from build123d import *

# Parameters (mm, degrees)
BOSS_EXTRUDE1_DEPTH     = 22.225
CUT_EXTRUDE3_DEPTH      = 155.828053821
CUT_EXTRUDE3_DEPTH_BACK = 155.828053821
BOSS_EXTRUDE3_DEPTH     = 12.7
SKETCH10_W              = 31.75
SKETCH10_H              = 3.175
CUT_EXTRUDE5_DEPTH      = 12.7
CUT_EXTRUDE4_REACH      = 158.104
SKETCH9_R               = 3.175
BOSS_EXTRUDE6_DEPTH     = 3.175
CUT_EXTRUDE8_REACH      = 139.445
BOSS_EXTRUDE7_DEPTH     = 12.7


with BuildPart() as part:
    # Sketch1 → Boss-Extrude1 (new body)
    with BuildSketch(Plane(origin=(0, 0, 0), x_dir=(1, 0, 0), z_dir=(0, 1, 0))):
        with BuildLine():
            Line((-15.875, 0), (-15.875, 34.925))
            Line((-15.875, 34.925), (-63.5, 34.925))
            Line((-63.5, 34.925), (-63.5, -68.511279424))
            ThreePointArc((-63.5, -68.511279424), (0, -85.725), (63.5, -68.511279424))
            Line((63.5, -68.511279424), (63.5, 34.925))
            Line((63.5, 34.925), (15.875, 34.925))
            Line((15.875, 34.925), (15.875, 0))
            Line((15.875, 0), (-15.875, 0))
        make_face()
        with BuildLine():
            ThreePointArc((34.925, -77.468283771), (0, -82.55), (-34.925, -77.468283771))
            Line((-34.925, -77.468283771), (-34.925, -3.175))
            Line((-34.925, -3.175), (34.925, -3.175))
            Line((34.925, -3.175), (34.925, -77.468283771))
        make_face(mode=Mode.SUBTRACT)
        with BuildLine():
            Line((-38.1, 0), (-38.1, -76.477264852))
            ThreePointArc((-38.1, -76.477264852), (-49.455952678, -72.128120752), (-60.325, -66.675))
            Line((-60.325, -66.675), (-60.325, 28.575))
            Line((-60.325, 28.575), (-38.1, 28.575))
            Line((-38.1, 28.575), (-38.1, 0))
        make_face(mode=Mode.SUBTRACT)
        with BuildLine():
            ThreePointArc((60.325, -66.675), (49.455952678, -72.128120752), (38.1, -76.477264852))
            Line((38.1, -76.477264852), (38.1, 0))
            Line((38.1, 0), (38.1, 28.575))
            Line((38.1, 28.575), (60.325, 28.575))
            Line((60.325, 28.575), (60.325, -66.675))
        make_face(mode=Mode.SUBTRACT)
    extrude(amount=BOSS_EXTRUDE1_DEPTH)

    # Sketch3 → Cut-Extrude3 (cut, two sides: drawn at the far end of the back side and taken through both)
    with BuildSketch(Plane.ZY.offset(63.5).offset(-CUT_EXTRUDE3_DEPTH_BACK)):
        Polygon((-229.576794349, -155.859828624), (-34.925, 6.35), (-15.875, 22.225), (178.776794349, 184.434828624), (-145.6428629, 573.738417323), (-553.996451598, 233.443760074), align=None)
    extrude(amount=CUT_EXTRUDE3_DEPTH + CUT_EXTRUDE3_DEPTH_BACK, mode=Mode.SUBTRACT)

    # Sketch7 → Boss-Extrude3 (add)
    with BuildSketch(Plane(origin=(-15.875, 0, 0), x_dir=(0, 0, -1), z_dir=(1, 0, 0))):
        with BuildLine():
            Line((34.925, 0), (34.925, 22.225))
            ThreePointArc((34.925, 22.225), (31.879952535, 28.318784481), (25.178488372, 29.542263716))
            Line((25.178488372, 29.542263716), (0, 22.225))
            Line((0, 22.225), (0, 0))
            Line((0, 0), (34.925, 0))
        make_face()
    boss_extrude3 = extrude(amount=-BOSS_EXTRUDE3_DEPTH)

    # Mirror1: Boss-Extrude3 across plane
    add(boss_extrude3.mirror(Plane(origin=(0, 0, 0), x_dir=(0, 0, 1), z_dir=(1, 0, 0))))

    # Sketch10 → Cut-Extrude5 (cut)
    with BuildSketch(Plane(origin=(0, 22.225, 0), x_dir=(1, 0, 0), z_dir=(0, 1, 0))):
        with Locations((0, -1.5875)):
            Rectangle(SKETCH10_W, SKETCH10_H)
    extrude(amount=-CUT_EXTRUDE5_DEPTH, mode=Mode.SUBTRACT)

    # Sketch8 → Cut-Revolve1 (revolve, cut)
    with BuildSketch(Plane(origin=(0, 26.545081967, -22.120901639), x_dir=(1, 0, 0), z_dir=(0, 0.7682212795973757, -0.6401843996644799)), mode=Mode.PRIVATE) as cut_revolve1_sk:
        Polygon((28.575, 6.748183757), (-28.575, 6.748183757), (-28.575, 9.748183757), (-26.425, 9.748183757), (-26.425, 10.748183757), (28.575, 10.748183757), align=None)
    revolve(cut_revolve1_sk.sketch.rotate(Axis((28.575, 22.225, -27.305), (-1, 0, 0)), 320.194428908), axis=Axis((28.575, 22.225, -27.305), (-1, 0, 0)), mode=Mode.SUBTRACT)

    # Sketch9 → Cut-Extrude4 (cut, up to next)
    with BuildSketch(Plane.ZY.offset(63.5), mode=Mode.PRIVATE) as cut_extrude4_sk1:
        with Locations((-15.875, 6.35)):
            Circle(SKETCH9_R)
    cut_extrude4_tool1 = extrude(cut_extrude4_sk1.sketch, amount=-CUT_EXTRUDE4_REACH, mode=Mode.PRIVATE) & part.part
    # Sketch9 → Cut-Extrude4 (cut, up to next)
    with BuildSketch(Plane.ZY.offset(63.5), mode=Mode.PRIVATE) as cut_extrude4_sk2:
        with Locations((55.245, 6.35)):
            Circle(SKETCH9_R)
    cut_extrude4_tool2 = extrude(cut_extrude4_sk2.sketch, amount=-CUT_EXTRUDE4_REACH, mode=Mode.PRIVATE) & part.part
    # Sketch9 → Cut-Extrude4 (cut, up to next)
    with BuildSketch(Plane.ZY.offset(63.5), mode=Mode.PRIVATE) as cut_extrude4_sk3:
        with Locations((19.685, 11.1125)):
            Circle(SKETCH9_R)
    cut_extrude4_tool3 = extrude(cut_extrude4_sk3.sketch, amount=-CUT_EXTRUDE4_REACH, mode=Mode.PRIVATE) & part.part
    cut_extrude4_1 = cut_extrude4_tool1.solids().sort_by_distance((-63.5, 6.35, -15.875))[0]
    add(cut_extrude4_1, mode=Mode.SUBTRACT)
    cut_extrude4_2 = cut_extrude4_tool2.solids().sort_by_distance((-63.5, 6.35, 55.245))[0]
    add(cut_extrude4_2, mode=Mode.SUBTRACT)
    cut_extrude4_3 = cut_extrude4_tool3.solids().sort_by_distance((-63.5, 11.1125, 19.685))[0]
    add(cut_extrude4_3, mode=Mode.SUBTRACT)
    cut_extrude4 = cut_extrude4_1 + cut_extrude4_2 + cut_extrude4_3  # Cut-Extrude4 as one shape, for the pattern or mirror that repeats it

    # Mirror10: Cut-Extrude4 across plane
    add(cut_extrude4.mirror(Plane(origin=(0, 0, 0), x_dir=(0, 0, 1), z_dir=(1, 0, 0))), mode=Mode.SUBTRACT)

    # Sketch16 → Boss-Extrude6 (add)
    with BuildSketch(Plane(origin=(-15.875, 0, 0), x_dir=(0, 0, -1), z_dir=(1, 0, 0))):
        with BuildLine():
            Line((-8.89, 29.845), (-3.175, 22.225))
            Line((-3.175, 22.225), (0, 22.225))
            Line((0, 22.225), (0, 0))
            Line((0, 0), (-3.175, 0))
            Line((-3.175, 0), (-26.242836689, 0))
            Line((-26.242836689, 0), (-31.317257994, 18.937998127))
            ThreePointArc((-31.317257994, 18.937998127), (-24.604350234, 33.645997919), (-8.89, 29.845))
        make_face()
    extrude(amount=-BOSS_EXTRUDE6_DEPTH)

    # Sketch17 → Cut-Extrude8 (cut, up to next)
    with BuildSketch(Plane.ZY.offset(38.1), mode=Mode.PRIVATE) as cut_extrude8_sk1:
        with BuildLine():
            Line((24.590354218, 5.1125), (14.779645782, 5.1125))
            ThreePointArc((14.779645782, 5.1125), (12.682179312, 7.792409277), (11.935, 11.1125))
            Line((11.935, 11.1125), (11.935, 22.225))
            Line((11.935, 22.225), (27.435, 22.225))
            Line((27.435, 22.225), (27.435, 11.1125))
            ThreePointArc((27.435, 11.1125), (26.687820688, 7.792409277), (24.590354218, 5.1125))
        make_face()
    cut_extrude8_tool1 = extrude(cut_extrude8_sk1.sketch, amount=-CUT_EXTRUDE8_REACH, mode=Mode.PRIVATE) & part.part
    cut_extrude8 = cut_extrude8_tool1.solids().sort_by_distance((-38.1, 13.958781, 19.685))[0]
    add(cut_extrude8, mode=Mode.SUBTRACT)

    # Mirror11: Cut-Extrude8 across plane
    add(cut_extrude8.mirror(Plane(origin=(0, 0, 0), x_dir=(0, 0, 1), z_dir=(1, 0, 0))), mode=Mode.SUBTRACT)

    # Sketch18 → Boss-Extrude7 (add)
    with BuildSketch(Plane(origin=(38.1, 0, 0), x_dir=(0, 0, -1), z_dir=(1, 0, 0))):
        with BuildLine():
            Line((-11.935, 22.225), (-11.935, 11.1125))
            ThreePointArc((-11.935, 11.1125), (-12.682179312, 7.792409277), (-14.779645782, 5.1125))
            Line((-14.779645782, 5.1125), (-24.590354218, 5.1125))
            ThreePointArc((-24.590354218, 5.1125), (-26.687820688, 7.792409277), (-27.435, 11.1125))
            Line((-27.435, 11.1125), (-27.435, 22.225))
            Line((-27.435, 22.225), (-29.975, 22.225))
            Line((-29.975, 22.225), (-29.975, 0))
            Line((-29.975, 0), (-9.395, 0))
            Line((-9.395, 0), (-9.395, 22.225))
            Line((-9.395, 22.225), (-11.935, 22.225))
        make_face()
    boss_extrude7 = extrude(amount=BOSS_EXTRUDE7_DEPTH)

    # Mirror12: Boss-Extrude7 across plane
    add(boss_extrude7.mirror(Plane(origin=(0, 0, 0), x_dir=(0, 0, 1), z_dir=(1, 0, 0))))


solid = part.part
Geometry: final body of the model. Coordinates: model frame, mm. A direction names the side the tool comes from. Give positions to 0.01 mm unless a question says otherwise; leave off trailing zeros. Write each loop counter-clockwise with the first axis right and the second up, starting at its lowest first coordinate (ties: lowest second). Pieces come first, ordered by that corner, then holes.
(1) Mould query, pull axis X, two halves, no side actions, for faces 1 (the cylindrical face through (-0.93, 10.96, 85.72)), 2 (the flat face through (-34, 6, -34.925)), 3 (the cylindrical face through (-42.75, 7.84, 12.66)), 4 (the flat face through (0, 5, 0)). Classes: released by +X, released by -X, zero draft, split by the parting line, or undercut.
(2) Ray query, line 1 (X direction, y = 2.5, z = -1) (3 decimals); line 2 (X direction, y = 21.5, z = 10) (3 decimals); line 3 (X direction, y = 12.5, z = 27) (3 decimals). Return the intervals inside material, ascending.
(3) Access query for faces 5 (the flat face through (-26.425, 19, -27)), 6 (the flat face through (-43, 17, 11.935)), 7 (the flat face through (-38.1, 11, -10)), 8 (the flat face through (32, 22.225, -2)). Directions: +Z, -Z, +X, -X, +Y, -Y. A direction counts if a zero-diameter tool reaches every point of the face in a straight line with its end or side. Return the directions, or none.
(4) Cut plane B-B, the plane x = 12. Return loops of the section in (y, z) (3 decimals), then the cut area to 3 significant figures.
(5) First-contact query: P1, Ø6, axis at x = 53.5, y = 4.5, coming from the +Z side; P2, Ø3, axis at x = -49.5, y = 23.5, coming from the -Z side (3 decimals); P3, Ø5.5, axis at y = 11.11, z = 19.68, coming from the +X side (3 decimals); P4, Ø6, axis at y = 27.5, z = 46, coming from the -X side. Flat tips, straight axial feed; report the tip coordinate or a pass-through.
(6) Cut plane C-C, the plane x = -47. Give the number of separate pieces and of enclosed holes in the cut face, then the cut area to 3 significant figures.
(7) Cut plane A-A, the plane z = 45. Return loops of the section in (x, y) (3 decimals).
Values follow:
1. face 1: split by the parting line
1. face 2: zero draft
1. face 3: undercut
1. face 4: undercut
2. line 1: x = -63.5 to -60.325, -38.1 to -15.875, 15.875 to 38.1, 60.325 to 63.5
2. line 2: x = -63.5 to -60.325, -50.8 to -34.925, -19.05 to -15.875, 34.925 to 50.8, 60.325 to 63.5
2. line 3: x = -63.5 to -60.325, -19.05 to -15.875, 60.325 to 63.5
3. face 5: +X
3. face 6: +Y
3. face 7: +Y, -Y
3. face 8: +Z, +X, +Y
4. outline: (0, 0) - (9.525, 0) - (9.525, 3.175) - (0, 3.175) - close; (0, 81.961) - (22.225, 81.961) - (22.225, 85.151) - (0, 85.151) - close
4. area: 101 mm2
5. P1: stops at z = 75.14
5. P2: stops at z = 9.395
5. P3: stops at x = -15.875
5. P4: passes through
6. separate pieces: 3
6. enclosed holes: 0
6. area: 336 mm2
7. outline: (-63.5, 0) - (-60.325, 0) - (-60.325, 22.225) - (-63.5, 22.225) - close; (-38.1, 0) - (-34.925, 0) - (-34.925, 22.225) - (-38.1, 22.225) - close; (34.925, 0) - (38.1, 0) - (38.1, 22.225) - (34.925, 22.225) - close; (60.325, 0) - (63.5, 0) - (63.5, 22.225) - (60.325, 22.225) - close
